```python
from build123d import *

# Parameters (mm, degrees)
F0_W     = 14
F0_H     = 39
F0_H_2   = 29
F1_DEPTH = 36
F2_W     = 14
F2_H     = 29
F3_DEPTH = 22
F4_W     = 14
F4_H     = 39
F5_DEPTH = 35
F6_W     = 17
F6_H     = 14
F7_DEPTH = 25
F8_W     = 12
F8_H     = 30
F9_DEPTH = 40


with BuildPart() as f1:
    # F0 (on Front) → F1 (new body)
    with BuildSketch(Plane.XZ):
        Polygon((-7, -34), (21, -34), (21, 34), (-7, 34), (-7, 5), align=None)
        with Locations((-14, -14.5)):
            Rectangle(F0_W, F0_H)
        with Locations((-14, 19.5)):
            Rectangle(F0_W, F0_H_2)
    extrude(amount=F1_DEPTH)

    # F2 (on face) → F3 (join)
    with BuildSketch(Plane.XZ.offset(36)):
        with Locations((-14, 19.5)):
            Rectangle(F2_W, F2_H)
    extrude(amount=F3_DEPTH)

    # F4 (on face) → F5 (join)
    with BuildSketch(Plane.XZ.offset(36)):
        with Locations((-14, -14.5)):
            Rectangle(F4_W, F4_H)
    extrude(amount=F5_DEPTH)

    # F6 (on face) → F7 (cut)
    with BuildSketch(Plane(origin=(-21, 0, 0), x_dir=(0, -1, 0), z_dir=(-1, 0, 0))):
        with Locations((57.56289, -13)):
            Rectangle(F6_W, F6_H)
    extrude(amount=-F7_DEPTH, mode=Mode.SUBTRACT)

    # F8 (on face) → F9 (cut)
    with BuildSketch(Plane.XZ.offset(36)):
        with Locations((8, -3)):
            Rectangle(F8_W, F8_H)
    extrude(amount=-F9_DEPTH, mode=Mode.SUBTRACT)


solid = f1.part
```
Verification items for the finished model (mm, model axes). A direction names the side the tool comes from. Give positions to 0.01 mm unless a question says otherwise; leave off trailing zeros. Write each loop counter-clockwise with the first axis right and the second up, starting at its lowest first coordinate (ties: lowest second). Pieces come first, ordered by that corner, then holes. Notation, with made-up numbers: (35.5, 21) - (39.5, 21) arc R9 cw to (39.5, 27) - close; hole circle Ø1 at (9, 38.5). An arc over 180 degrees is marked (long way). Put each result on its own line as item: value.
Q1. Mould release check, pull along Y, two halves, no side actions. Record for faces 5 (the face through (-14, -57, -6)), 6 (the face through (1, -36, 0)), 7 (the face through (21, -18, 0)): released by +Y, released by -Y, zero draft, split by the parting line, or undercut.
Result:
face 5: undercut
face 6: released by -Y
face 7: zero draft
Q2. Scan lines: probe 1 along Y at (x, z) = (-17, -16); probe 2 along Z at (x, y) = (5, -12); probe 3 along X at (y, z) = (-19, -13.5). Record each from-to range of solid material in increasing order. Write a range as from..to.
Result:
probe 1: -71..-66.06, -49.06..0
probe 2: -34..-18, 12..34
probe 3: -21..2, 14..21
Q3. Depth check by flat-ended pin: P1, Ø11, axis at x = -11.5, z = -15, coming from the +Y side; P2, Ø12, axis at x = 3, z = -4, coming from the -Y side; P3, Ø6, axis at y = -48.5, z = 24, coming from the +X side; P4, Ø4, axis at x = -14.5, y = -67.5, coming from the +Z side. Enter the tip coordinate at first touch or a pass-through.
Result:
P1: y = 0
P2: y = -36
P3: x = -7
P4: z = 5
Q4. Set-up check for faces 1 (the face through (-14, -58, 20)), 2 (the face through (-14, -57, -20)), 3 (the face through (8, -18, -18)), 4 (the face through (-7, -49, 0)): record each of +Z, -Z, +X, -X, +Y, -Y from which the full face is reachable in a straight line by a thin tool's end or side.
Result:
face 1: +Z, +X, -X, -Y
face 2: +X, -X
face 3: +Y, -Y
face 4: +Z, -Z, +X, -Y
Q5. Section check C-C on z = -2. Record the cut outline in (x, y), and give its area (3 significant figures).
Result:
outline: (-21, -71) - (-7, -71) - (-7, -36) - (2, -36) - (2, 0) - (-21, 0) - close; (14, -36) - (21, -36) - (21, 0) - (14, 0) - close
area: 1,570 mm2
Q6. Section check A-A on x = 10. Record the cut outline in (y, z).
Result:
outline: (-36, -34) - (0, -34) - (0, -18) - (-36, -18) - close; (-36, 12) - (0, 12) - (0, 34) - (-36, 34) - close
Q7. Section check D-D on y = -23. Record the cut outline in (x, z).
Result:
outline: (-21, -34) - (21, -34) - (21, 34) - (-21, 34) - close; hole (2, -18) - (14, -18) - (14, 12) - (2, 12) - close
Q8. Section check B-B on y = -59. Record the cut outline in (x, z), and give its area (3 significant figures).
Result:
outline: (-21, -34) - (-7, -34) - (-7, -20) - (-21, -20) - close; (-21, -6) - (-7, -6) - (-7, 5) - (-21, 5) - close
area: 350 mm2
